Could you check a few things on this model? Use its own coordinates, in mm. Face numbers are marked on the shaded views. A direction names the side the tool comes from. Round coordinates to 2 decimals unless told otherwise and drop trailing zeros. Order: outer loops, then holes, each group sorted by start corner. A loop starts at its lowest first (then second) coordinate and runs counter-clockwise, first axis right, second up. Notation, with made-up numbers: (70.5, 2.5) - (119.5, 2.5) arc R24 cw to (119.5, 28.5) - close; hole circle Ø7 at (-23.75, 74.25). An arc over 180 degrees is marked (long way). Return JSON: item names as keys, results as strings. Group by question number.
from build123d import *

# Parameters (mm, degrees)
SKETCH1_W           = 12
SKETCH1_H           = 15
BOSS_EXTRUDE1_DEPTH = 13
CUT_EXTRUDE1_DEPTH  = 8


with BuildPart() as part:
    # Sketch1 → Boss-Extrude1 (new body)
    with BuildSketch(Plane.XY):
        Rectangle(SKETCH1_W, SKETCH1_H)
    extrude(amount=BOSS_EXTRUDE1_DEPTH)

    # Sketch2 → Cut-Extrude1 (cut)
    with BuildSketch(Plane.XY):
        Polygon((1.331268312, 6.434952315), (-1.331268312, 6.434952315), (-1.331268312, 5.674031135), (-2.949806732, 5.674031135), (-2.949806732, 4.197823958), (-5.051214446, 4.197823958), (-5.051214446, -7.5), (5.051214446, -7.5), (5.051214446, 4.197823958), (2.949806732, 4.197823958), (2.949806732, 5.674031135), (1.331268312, 5.674031135), align=None)
    extrude(amount=CUT_EXTRUDE1_DEPTH, mode=Mode.SUBTRACT)


solid = part.part
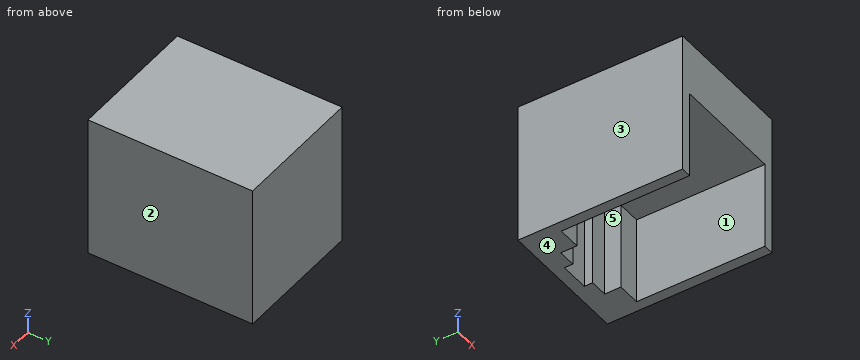
1) I want a section at D-D, the plane x = -4. List the corners of the cut face in (y, z) for me, plus the area to 3 significant figures.
2) Will these pins go through, and if not, where does the flat tip stop? pin 1 (0.5 mm diameter, centred on x = 2.5, z = 5.5, fed in from -Y); pin 2 (1.1 mm diameter, centred on x = -4, z = 5, fed in from -Y); pin 3 (1.3 mm diameter, centred on x = 0.5, z = 5.5, fed in from -Y); pin 4 (2 mm diameter, centred on x = 4.5, y = -1, fed in from -Z).
3) We'd pull the mould along X, two halves only. Please class the marked faces 3, 4 and 5: +X half, -X half, draft (parallel to the pull), parting line (faces both ways), or undercut.
4) If I drill on line 1 along X through (y, z) = (-5.75, 0.75); line 2 along Y through (x, z) = (-1.25, 3); line 3 along Z through (x, y) = (3.75, -0.5), over which ranges is the centre line in solid material (lowest first)? Write a range as from..to.
5) I want a section at C-C, the plane y = -2. List the corners of the cut face in (x, z) for me.
6) I want a section at B-B, the plane z = 7. List the corners of the cut face in (x, y) for me.
7) For the marked faces 1 and 2, which set-ups out of +Z, -Z, +X, -X, +Y, -Y let a thin tool reach every point of the face, with its end or its side?
8) I want a section at A-A, the plane x = -0.75. List the corners of the cut face in (y, z) for me, plus the area to 3 significant figures.
Outcome:
{
 "1": {"outline": "(-7.5, 8) - (4.2, 8) - (4.2, 0) - (7.5, 0) - (7.5, 13) - (-7.5, 13) - close", "area": "101 mm^2"},
 "2": {"pin 1": "y = 5.67", "pin 2": "y = 4.2", "pin 3": "y = 6.43", "pin 4": "z = 0"},
 "3": {"face 3": "-X half", "face 4": "draft", "face 5": "undercut"},
 "4": {"line 1": "-6..-5.05, 5.05..6", "line 2": "6.43..7.5", "line 3": "8..13"},
 "5": {"outline": "(-6, 0) - (-5.05, 0) - (-5.05, 8) - (5.05, 8) - (5.05, 0) - (6, 0) - (6, 13) - (-6, 13) - close"},
 "6": {"outline": "(-6, -7.5) - (-5.05, -7.5) - (-5.05, 4.2) - (-2.95, 4.2) - (-2.95, 5.67) - (-1.33, 5.67) - (-1.33, 6.43) - (1.33, 6.43) - (1.33, 5.67) - (2.95, 5.67) - (2.95, 4.2) - (5.05, 4.2) - (5.05, -7.5) - (6, -7.5) - (6, 7.5) - (-6, 7.5) - close"},
 "7": {"face 1": "-Z, -Y", "face 2": "+Z, -Z, +X, +Y, -Y"},
 "8": {"outline": "(-7.5, 8) - (6.43, 8) - (6.43, 0) - (7.5, 0) - (7.5, 13) - (-7.5, 13) - close", "area": "83.5 mm^2"}
}
